Geometry check sheet. Reference: the model listing, model coordinates, mm. A direction names the side the tool comes from. Round coordinates to 2 decimals unless told otherwise and drop trailing zeros. Order: outer loops, then holes, each group sorted by start corner. A loop starts at its lowest first (then second) coordinate and runs counter-clockwise, first axis right, second up. Notation, with made-up numbers: (83, -39.75) -> (92, -39.75) arc R16 ccw to (92, -25.75) -> close; hole circle Ø6 at (-25.5, 8). An arc over 180 degrees is marked (long way). Answer as a JSON object with one key per item and string values. Group by question number.
from build123d import *

# Parameters (mm, degrees)
BOSS_EXTRUDE1_DEPTH  = 1.5875
FILLET1_R            = 2.54
M4_CLEARANCE_HOLE1_D = 4.5
FILLET2_R            = 6.35
FILLET3_R            = 12.7
FILLET4_R            = 3.175


with BuildPart() as part:
    # Sketch1 → Boss-Extrude1 (new body)
    with BuildSketch(Plane(origin=(0, 0, 0), x_dir=(0, 0, -1), z_dir=(1, 0, 0))):
        with BuildLine():
            Line((832.226267655, 544.132439772), (843.624269089, 544.132439772))
            Line((843.624269089, 544.132439772), (847.764493389, 544.132439772))
            Line((847.764493389, 544.132439772), (865.776854812, 544.132439772))
            Line((865.776854812, 544.132439772), (869.917079112, 544.132439772))
            Line((869.917079112, 544.132439772), (870.226267655, 544.132439772))
            Line((870.226267655, 544.132439772), (870.226267655, 554.132439772))
            ThreePointArc((870.226267655, 554.132439772), (869.347587998, 556.253760115), (867.226267655, 557.132439772))
            Line((867.226267655, 557.132439772), (832.226267655, 557.132439772))
            ThreePointArc((832.226267655, 557.132439772), (830.812054092, 556.546653334), (830.226267655, 555.132439772))
            Line((830.226267655, 555.132439772), (830.226267655, 546.132439772))
            ThreePointArc((830.226267655, 546.132439772), (830.812054092, 544.718226209), (832.226267655, 544.132439772))
        make_face()
        with BuildLine():
            Line((847.764493389, 544.132439772), (863.880128333, 483.796291029))
            add(Edge.make_bspline(
                [(863.880128333, 483.796291029), (865.574478469, 486.592797057), (868.03804251, 488.340736874), (870.62475601, 489.202974707)],
                knots=[0.867438588, 0.867438588, 0.867438588, 0.867438588, 1, 1, 1, 1], degree=3, weights=[0.610334575, 0.693362976, 0.82325145, 1]))
            add(Edge.make_bspline(
                [(870.62475601, 489.202974707), (873.662795809, 490.21565464), (877.265107333, 490.148897283), (880.706436997, 488.236814526)],
                knots=[0, 0, 0, 0, 0.151032869, 0.151032869, 0.151032869, 0.151032869], degree=3, weights=[1, 0.798622841, 0.658074822, 0.578355943]))
            Line((880.706436997, 488.236814526), (865.776854812, 544.132439772))
            Line((865.776854812, 544.132439772), (847.764493389, 544.132439772))
        make_face()
    extrude(amount=-BOSS_EXTRUDE1_DEPTH)

    # Fillet1
    fillet1_edges = [part.edges().sort_by_distance(p)[0] for p in [
        (-0.79375, 488.236814526, -880.706436997),
        (-0.79375, 483.796291029, -863.880128333),
    ]]
    fillet(fillet1_edges, radius=FILLET1_R)

    # M4 Clearance Hole1 (through all)
    with Locations(Plane.ZY.offset(1.5875)):
        with Locations((-860.226267655, 550.632439772), (-840.226267655, 550.632439772)):
            Hole(M4_CLEARANCE_HOLE1_D / 2)

    # Fillet2
    # the kernel refuses this fillet: 6.35 mm, written as the material it adds along each edge
    with BuildSketch(Plane(origin=(0, 544.132439772, -865.776854812), x_dir=(0, -0.9661312310415323, -0.25805124376017496), z_dir=(-1, 0, 0))) as fillet2_piece_1:
        with BuildLine():
            CenterArc((7.157730316, -6.35), FILLET2_R, 90, 71.153326235)
            Line((1.148176518, -4.298716707), (1.027985442, -4.257691041))
            ThreePointArc((1.027985442, -4.257691041), (0.451389593, -2.182130862), (-0.122698666, -0.032772508))
            Line((-0.122698666, -0.032772508), (0, 0.127))
            Line((0, 0.127), (7.157730316, 0.127))
            Line((7.157730316, 0.127), (7.157730316, 0))
        make_face()
    extrude(amount=1.5875)

    # Fillet3
    fillet3_edges = [part.edges().sort_by_distance(p)[0] for p in [
        (-0.79375, 544.132439772, -847.764493389),
    ]]
    fillet(fillet3_edges, radius=FILLET3_R)

    # Fillet4
    fillet4_edges = [part.edges().sort_by_distance(p)[0] for p in [
        (-0.79375, 544.132439772, -870.226267655),
    ]]
    fillet(fillet4_edges, radius=FILLET4_R)


solid = part.part
Item 1: Sectioned sample at A-A, the plane z = -841.5. Enter the section's corners in (x, y), then the cut area to 3 significant figures.
Item 2: Depth check by flat-ended pin: pin 1 Ø6 at (y, z) = (550.63, -840.23) entering from +X. Enter the tip coordinate at first touch or a pass-through.
Item 3: Sectioned sample at B-B, the plane y = 547.5. Enter the section's corners in (x, z).
Item 4: Set-up check for faces 1 (the flat face through (-1, 550, -870.226)), 2 (the flat face through (-0.783, 514.714, -873.635)), 3 (the cylindrical face through (-0.78, 550.73, -837.98)): record each of +Z, -Z, +X, -X, +Y, -Y from which the full face is reachable in a straight line by a thin tool's end or side.
Item 5: Mould release check, pull along Y, two halves, no side actions. Record for faces 4 (the flat face through (-1, 544.132, -835)), 5 (the cylindrical face through (-0.8, 556.2, -869.4)), 6 (the flat face through (-1, 551, -830.226)), 7 (the cylindrical face through (-0.783, 540.469, -867.617)): pulls with the +Y half, pulls with the -Y half, needs draft (parallel to the pull), parting line crosses it, or undercut.
Item 6: Sectioned sample at C-C, the plane x = -1.25. Count the separate pieces of the cut face and the enclosed holes in it, then the cut area to 3 significant figures.
Item 7: Thickness scan on L1, parallel to Z at x = -1.5, y = 551; L2, parallel to Z at x = -0.4, y = 547; L3, parallel to Y at x = -1, z = -837.5. Record the ranges inside material, lowest first.
Item 8: Sectioned sample at D-D, the plane z = -848. Enter the section's corners in (x, y).
Result:
{
 "1": {"outline": "(-1.59, 543.64) -> (0, 543.64) -> (0, 548.78) -> (-1.59, 548.78) -> close; (-1.59, 552.49) -> (0, 552.49) -> (0, 557.13) -> (-1.59, 557.13) -> close", "area": "15.5 mm2"},
 "2": {"pin 1": "stops at x = 0"},
 "3": {"outline": "(-1.59, -870.23) -> (0, -870.23) -> (0, -830.23) -> (-1.59, -830.23) -> close"},
 "4": {"face 1": "-Z, +X, -X, +Y", "face 2": "-Z, +X, -X", "face 3": "+X, -X"},
 "5": {"face 4": "pulls with the -Y half", "face 5": "pulls with the +Y half", "face 6": "needs draft", "face 7": "undercut"},
 "6": {"separate pieces": "1", "enclosed holes": "2", "area": "1,510 mm2"},
 "7": {"L1": "z = -870.23 to -862.45, -858.01 to -842.45, -838.01 to -830.23", "L2": "z = -870.23 to -830.23", "L3": "y = 544.13 to 557.13"},
 "8": {"outline": "(-1.59, 539.28) -> (0, 539.28) -> (0, 557.13) -> (-1.59, 557.13) -> close"}
}
